Geometry check sheet. Reference: the model listing, model coordinates, mm. A direction names the side the tool comes from. Round coordinates to 2 decimals unless told otherwise and drop trailing zeros. Order: outer loops, then holes, each group sorted by start corner. A loop starts at its lowest first (then second) coordinate and runs counter-clockwise, first axis right, second up.
```python
from build123d import *

# Parameters (mm, degrees)
SKETCH1_R           = 3
SKETCH1_W           = 10
SKETCH1_H           = 3
BOSS_EXTRUDE1_DEPTH = 3


with BuildPart() as part:
    # Sketch1 → Boss-Extrude1 (new body)
    with BuildSketch(Plane.XY):
        Polygon((-31.361502347, 21.305164319), (33.638497653, 21.305164319), (33.638497653, 17.769219388), (63.638497653, 17.769219388), (63.638497653, 21.305164319), (128.638497653, 21.305164319), (128.638497653, 11.427031749), (131.638497653, 11.427031749), (131.638497653, -13.572968251), (128.638497653, -13.572968251), (128.638497653, -24.694835681), (-31.361502347, -24.694835681), (-31.361502347, -13.572968251), (-34.361502347, -13.572968251), (-34.361502347, 11.427031749), (-31.361502347, 11.427031749), align=None)
        with Locations((48.638497653, 10.769219388)):
            Circle(SKETCH1_R, mode=Mode.SUBTRACT)
        with Locations((-1.361502347, -20.072968251)):
            Rectangle(SKETCH1_W, SKETCH1_H, mode=Mode.SUBTRACT)
        with Locations((-21.361502347, -20.072968251)):
            Rectangle(SKETCH1_W, SKETCH1_H, mode=Mode.SUBTRACT)
        with Locations((18.638497653, -20.072968251)):
            Rectangle(SKETCH1_W, SKETCH1_H, mode=Mode.SUBTRACT)
        with Locations((38.638497653, -20.072968251)):
            Rectangle(SKETCH1_W, SKETCH1_H, mode=Mode.SUBTRACT)
        with Locations((58.638497653, -20.072968251)):
            Rectangle(SKETCH1_W, SKETCH1_H, mode=Mode.SUBTRACT)
        with Locations((78.638497653, -20.072968251)):
            Rectangle(SKETCH1_W, SKETCH1_H, mode=Mode.SUBTRACT)
        with Locations((98.638497653, -20.072968251)):
            Rectangle(SKETCH1_W, SKETCH1_H, mode=Mode.SUBTRACT)
        with Locations((118.638497653, -20.072968251)):
            Rectangle(SKETCH1_W, SKETCH1_H, mode=Mode.SUBTRACT)
    extrude(amount=BOSS_EXTRUDE1_DEPTH)


solid = part.part
```
(1) Depth check by flat-ended pin: P1, Ø1.5, axis at y = -19.5, z = 1, coming from the +X side; P2, Ø1.5, axis at y = -21, z = 1, coming from the -X side. Enter the tip coordinate at first touch or a pass-through.
Returned:
P1: stops at x = 128.64
P2: stops at x = -31.36
(2) Sectioned sample at C-C, the plane x = -1. Record the cut outline in (y, z), and give its area (3 significant figures).
Returned:
outline: (-24.69, 0) - (-21.57, 0) - (-21.57, 3) - (-24.69, 3) - close; (-18.57, 0) - (21.31, 0) - (21.31, 3) - (-18.57, 3) - close
area: 129 mm2
(3) Set-up check for faces 4 (the flat face through (113.638, -20, 1)), 5 (the flat face through (50, -1, 3)), 6 (the flat face through (-31.362, 16, 1)), 7 (the flat face through (63.638, 20, 1)): record each of +Z, -Z, +X, -X, +Y, -Y from which the full face is reachable in a straight line by a thin tool's end or side.
Returned:
face 4: +Z, -Z
face 5: +Z, +X, -X, +Y, -Y
face 6: +Z, -Z, -X, +Y
face 7: +Z, -Z, +Y
(4) Draft check along Y on faces 1 (the flat face through (-1, -18.573, 1)), 2 (the flat face through (130, -13.573, 1)), 3 (the flat face through (1, 21.305, 1)). Enter one of: released by +Y, released by -Y, zero draft, split by the parting line, or undercut.
Returned:
face 1: undercut
face 2: released by -Y
face 3: released by +Y
(5) Sectioned sample at B-B, the plane y = -20. Give the number of separate pieces and of enclosed holes in the cut face, and give its area (3 significant figures).
Returned:
separate pieces: 9
enclosed holes: 0
area: 240 mm2
(6) Sectioned sample at A-A, the plane x = 56.5. Record the cut outline in (y, z), and give its area (3 significant figures).
Returned:
outline: (-24.69, 0) - (-21.57, 0) - (-21.57, 3) - (-24.69, 3) - close; (-18.57, 0) - (17.77, 0) - (17.77, 3) - (-18.57, 3) - close
area: 118 mm2
(7) Material ranges on line 1 (Y direction, x = -24, z = 0.75); line 2 (Y direction, x = 63.5, z = 1.45); line 3 (X direction, y = 19.5, z = 1.45), recorded low to high.
Returned:
line 1: y = -24.69 to -21.57, -18.57 to 21.31
line 2: y = -24.69 to -21.57, -18.57 to 17.77
line 3: x = -31.36 to 33.64, 63.64 to 128.64
